Verification items for the finished model (mm, model axes). Face numbers are marked on the shaded views. A direction names the side the tool comes from. Coordinates: 2 decimals unless noted, no trailing zeros. Order: outer loops, then holes, each group sorted by start corner. A loop starts at its lowest first (then second) coordinate and runs counter-clockwise, first axis right, second up. Notation, with made-up numbers: M 22,13 L 40,13 A17 ccw 40,22 Z; hole C -1.75,54 d4. An arc over 180 degrees is marked long. Return JSON: item names as keys, results as strings.
```python
from build123d import *

# Parameters (mm, degrees)
F0_R     = 1.5262492047
F0_R_2   = 5.564877875
F0_R_3   = 2.6305534458
F1_DEPTH = 6.35


# Not quite as in the source:
# - a feature names something its author has since deleted; it is built from what else it names


with BuildPart() as f1:
    # F0 (on Top) → F1 (new body)
    with BuildSketch(Plane.XY):
        with BuildLine():
            Line((-18.5164521814, -21.5775697793), (0, -54.5748323202))
            Line((0, -54.5748323202), (19.7828651091, -19.6195188363))
            Line((19.7828651091, -19.6195188363), (22.6427465677, -14.5662541873))
            Line((22.6427465677, -14.5662541873), (30.8864787221, 0))
            ThreePointArc((30.8864787221, 0), (2.0232479541, 30.1763499671), (-30.3273923907, 3.7730498517))
            ThreePointArc((-30.3273923907, 3.7730498517), (-30.5341463656, 1.8911023526), (-30.6247305125, 0))
            Line((-30.6247305125, 0), (-19.4482157174, -19.9171196174))
            Line((-19.4482157174, -19.9171196174), (-18.5164521814, -21.5775697793))
        make_face()
        Polygon((22.1472843044, -0.5254783843), (0.0272358089, -39.6104756875), (-21.9053558016, -0.5254783843), (0.1308741048, -0.5254783843), align=None, mode=Mode.SUBTRACT)
        with Locations((-16.2284877151, 12.1713718399)):
            Circle(F0_R, mode=Mode.SUBTRACT)
        with Locations((0, 15.3123699129)):
            Circle(F0_R_2, mode=Mode.SUBTRACT)
        with Locations((18.8459847122, 12.1713718399)):
            Circle(F0_R_3, mode=Mode.SUBTRACT)
        Polygon((22.6427465677, -14.5662541873), (19.7828651091, -19.6195188363), (19.7828651091, -38.1040237844), (22.6427465677, -38.1040237844), align=None)
        Polygon((-25.7906284703, -25.6594822484), (-18.5164521814, -21.5775697793), (-19.4482157174, -19.9171196174), (-26.7223920062, -23.9990320865), align=None)
        with BuildLine():
            Line((-49.3409076612, 0), (-30.6247305125, 0))
            ThreePointArc((-30.6247305125, 0), (-30.5341463656, 1.8911023526), (-30.3273923907, 3.7730498517))
            Line((-30.3273923907, 3.7730498517), (-49.3409076612, 3.7730498517))
            Line((-49.3409076612, 3.7730498517), (-49.3409076612, 0))
        make_face()
    extrude(amount=F1_DEPTH)


solid = f1.part
```
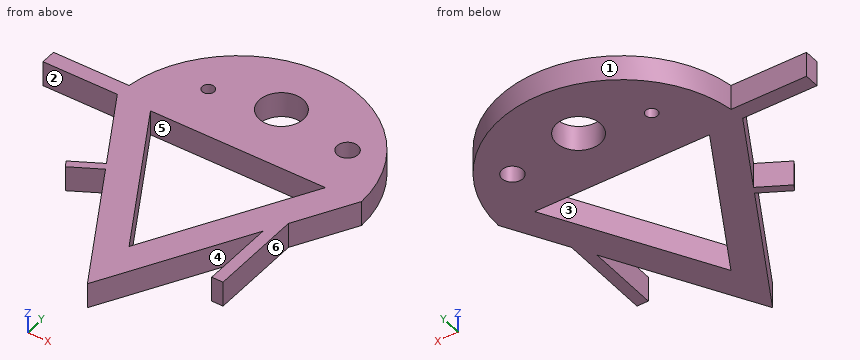
Q1. Material ranges on line 1 along X through (y, z) = (-26, 1.5); line 2 along X through (y, z) = (12.5, 0.75); line 3 along X through (y, z) = (-32, 6.25), recorded low to high.
Values:
{"line 1": "-16.03 to -7.61, 7.73 to 16.17, 19.78 to 22.64", "line 2": "-27.74 to -17.72, -14.74 to -4.8, 4.8 to 16.24, 21.46 to 28", "line 3": "-12.67 to -4.24, 4.33 to 12.78, 19.78 to 22.64"}
Q2. Cross-section at A-A, the plane x = 1. Record the boundary of the cut face in (y, z).
Values:
{"outline": "M -52.81,0 L -37.89,0 L -37.89,6.35 L -52.81,6.35 Z; M -0.53,0 L 9.84,0 L 9.84,6.35 L -0.53,6.35 Z; M 20.79,0 L 30.22,0 L 30.22,6.35 L 20.79,6.35 Z"}
Q3. Cross-section at D-D, the plane z = 2.75. Record the boundary of the cut face in (x, y), and give its area (3 significant figures).
Values:
{"outline": "M -49.34,0 L -30.62,0 L -19.45,-19.92 L -26.72,-24 L -25.79,-25.66 L -18.52,-21.58 L 0,-54.57 L 19.78,-19.62 L 19.78,-38.1 L 22.64,-38.1 L 22.64,-14.57 L 30.89,0 A30.76 ccw -30.33,3.77 L -49.34,3.77 Z; hole M -21.91,-0.53 L 0.03,-39.61 L 22.15,-0.53 Z; hole C -16.23,12.17 d3.05; hole C 0,15.31 d11.13; hole C 18.85,12.17 d5.26", "area": "2,290 mm^2"}
Q4. Tool access check on the marked faces 4, 5 and 6. Record the directions out of +Z, -Z, +X, -X, +Y, -Y that give a thin tool (end or side, any length) a straight path to the whole face; none if there is none.
Values:
{"face 4": "+Z, -Z, -Y", "face 5": "+Z, -Z", "face 6": "+Z, -Z, +X, -Y"}
Q5. Cross-section at B-B, the plane y = -30. Record the boundary of the cut face in (x, z).
Values:
{"outline": "M -13.79,0 L -5.37,0 L -5.37,6.35 L -13.79,6.35 Z; M 5.47,0 L 13.91,0 L 13.91,6.35 L 5.47,6.35 Z; M 19.78,0 L 22.64,0 L 22.64,6.35 L 19.78,6.35 Z"}
Q6. Draft check along Y on the marked faces 1, 2 and 3. Enter one of: pulls with the +Y half, pulls with the -Y half, needs draft (parallel to the pull), parting line crosses it, or undercut.
Values:
{"face 1": "pulls with the +Y half", "face 2": "pulls with the -Y half", "face 3": "undercut"}
Q7. Cross-section at C-C, the plane x = -7.5. Record the boundary of the cut face in (y, z).
Values:
{"outline": "M -41.21,0 L -26.2,0 L -26.2,6.35 L -41.21,6.35 Z; M -0.53,0 L 29.27,0 L 29.27,6.35 L -0.53,6.35 Z"}
Q8. Go/stop test with flat-tipped pins: pin 1 (3 mm diameter, centred on x = -39, z = 2.5, fed in from -Y); pin 2 (1.9 mm diameter, centred on y = -30, z = 4.5, fed in from -X); pin 3 (2.5 mm diameter, centred on x = 20.5, z = 3.5, fed in from -Y). Record where each tip stops, or that it passes through.
Values:
{"pin 1": "y = 0", "pin 2": "x = -14.32", "pin 3": "y = -38.1"}
